from build123d import *

# Parameters (mm, degrees)
BOSS_EXTRU_1_DEPTH              = 12
ENL_V_MAT_EXTRU_1_DEPTH         = 119.989845505
ENL_V_MAT_EXTRU_2_DEPTH         = 11
ENL_V_MAT_EXTRU_3_DEPTH         = 9.5
BOSS_EXTRU_6_DEPTH              = 2.2
BOSS_EXTRU_8_DEPTH              = 1.5
BOSS_EXTRU_7_DEPTH              = 3
BOSS_EXTRU_7_DIRECTION_2_REACH  = 102.687
CHANFREIN3_SIZE                 = 2.2
ENL_V_DE_MAT_EXTRU_MINCE1_DEPTH = 1.6
ENL_V_DE_MAT_EXTRU_MINCE1_DRAFT = 10
ENL_V_MAT_EXTRU_10_DEPTH        = 11


with BuildPart() as part:
    # Esquisse1 → Boss.-Extru.1 (new body)
    with BuildSketch(Plane(origin=(0, 0, 0), x_dir=(1, 0, 0), z_dir=(0, 1, 0))):
        Polygon((-77.5, -44.744645862), (77.5, -44.744645862), (0, 89.489291724), align=None)
    extrude(amount=BOSS_EXTRU_1_DEPTH)

    # Esquisse2 → Enlèv. mat.-Extru.1 (cut, through all)
    with BuildSketch(Plane(origin=(0, 12, 0), x_dir=(1, 0, 0), z_dir=(0, 1, 0))):
        Polygon((-9.237604307, 73.489291724), (9.237604307, 73.489291724), (0, 89.489291724), align=None)
        Polygon((77.5, -44.744645862), (68.262395693, -28.744645862), (59.024791386, -44.744645862), align=None)
        Polygon((-77.5, -44.744645862), (25.833333333, -44.744645862), (-25.833333333, 44.744645862), align=None)
    extrude(amount=-ENL_V_MAT_EXTRU_1_DEPTH, mode=Mode.SUBTRACT)

    # Esquisse3 → Enlèv. mat.-Extru.2 (cut)
    with BuildSketch(Plane(origin=(0, 12, 0), x_dir=(1, 0, 0), z_dir=(0, 1, 0))):
        with BuildLine():
            Line((59.313466521, -20.244645862), (12.124355653, 61.489291724))
            ThreePointArc((12.124355653, 61.489291724), (0, 68.489291724), (-12.124355653, 61.489291724))
            Line((-12.124355653, 61.489291724), (-21.791881449, 44.744645862))
            Line((-21.791881449, 44.744645862), (27.854059275, -41.244645862))
            Line((27.854059275, -41.244645862), (47.189110868, -41.244645862))
            ThreePointArc((47.189110868, -41.244645862), (59.313466521, -34.244645862), (59.313466521, -20.244645862))
        make_face()
    extrude(amount=-ENL_V_MAT_EXTRU_2_DEPTH, mode=Mode.SUBTRACT)

    # Esquisse4 → Enlèv. mat.-Extru.3 (cut)
    with BuildSketch(Plane(origin=(0, 12, 0), x_dir=(1, 0, 0), z_dir=(0, 1, 0))):
        Polygon((37.068911087, 18.284054341), (34.368911087, 22.960591521), (37.4, 24.710591521), (40.1, 20.034054341), align=None)
    extrude(amount=-ENL_V_MAT_EXTRU_3_DEPTH, mode=Mode.SUBTRACT)

    # Esquisse14 → Boss.-Extru.6 (add)
    with BuildSketch(Plane(origin=(0, 1, 0), x_dir=(1, 0, 0), z_dir=(0, 1, 0))):
        Polygon((32.699295844, 24.65244995), (37.699295844, 15.992195912), (35.967245037, 14.992195912), (30.967245037, 23.65244995), align=None)
    extrude(amount=BOSS_EXTRU_6_DEPTH)

    # Esquisse19 → Boss.-Extru.8 (add)
    with BuildSketch(Plane(origin=(0, 2.5, 0), x_dir=(1, 0, 0), z_dir=(0, 1, 0))):
        Polygon((34.368911087, 22.960591521), (37.068911087, 18.284054341), (36.549295844, 17.984054341), (33.849295844, 22.660591521), align=None)
    extrude(amount=-BOSS_EXTRU_8_DEPTH)

    # Esquisse15 → Boss.-Extru.7 (add)
    with BuildSketch(Plane(origin=(0, 3.2, 0), x_dir=(1, 0, 0), z_dir=(0, 1, 0))):
        Polygon((35.159103466, 20.991938173), (35.759103466, 19.952707689), (33.767245037, 18.802707689), (33.167245037, 19.841938173), align=None)
    extrude(amount=BOSS_EXTRU_7_DEPTH)

    # Boss.-Extru.7 direction 2: up to this face of the body (flat: up to its plane)
    boss_extru_7_direction_2_end = Plane(part.part.faces().sort_by_distance((19.594473703, 1, -11.312874667))[0])
    # Esquisse15 → Boss.-Extru.7 direction 2 (add, up to the picked face)
    with BuildSketch(Plane(origin=(0, 3.2, 0), x_dir=(1, 0, 0), z_dir=(0, 1, 0)), mode=Mode.PRIVATE) as boss_extru_7_direction_2_sk1:
        Polygon((35.159103466, 20.991938173), (35.759103466, 19.952707689), (33.767245037, 18.802707689), (33.167245037, 19.841938173), align=None)
    boss_extru_7_direction_2_tool1 = split(extrude(boss_extru_7_direction_2_sk1.sketch, amount=-BOSS_EXTRU_7_DIRECTION_2_REACH, mode=Mode.PRIVATE), bisect_by=boss_extru_7_direction_2_end, keep=Keep.BOTH, mode=Mode.PRIVATE)
    add(boss_extru_7_direction_2_tool1.solids().sort_by(Axis((34.463174, 3.2, -19.897323), (0, -1, 0)))[0])

    # Chanfrein3
    chanfrein3_edges = [part.edges().sort_by_distance(p)[0] for p in [
        (33.467245037, 1, -19.322322931),
        (36.833270441, 1, -15.492195912),
        (31.833270441, 1, -24.15244995),
    ]]
    chamfer(chanfrein3_edges, length=CHANFREIN3_SIZE - 0.0001)  # a hair under: the kernel refuses the full size


with BuildPart() as enl_v_de_mat_extru_mince1_tool:
    # Esquisse17 → Enlèv. de mat.-Extru.-Mince1 (with draft: the straight prism first)
    with BuildSketch(Plane(origin=(0, 12, 0), x_dir=(1, 0, 0), z_dir=(0, 1, 0))):
        Polygon((37.4, 24.710591521), (9.237604307, 73.489291724), (-9.237604307, 73.489291724), (-25.833333333, 44.744645862), (25.833333333, -44.744645862), (59.024791386, -44.744645862), (68.262395693, -28.744645862), (40.1, 20.034054341), (38.454551733, 19.084054341), (66.06846467, -28.744645862), (57.927825874, -42.844645862), (26.930298845, -42.844645862), (-23.63940231, 44.744645862), (-8.140638796, 71.589291724), (8.140638796, 71.589291724), (35.754551733, 23.760591521), align=None)
    extrude(amount=-ENL_V_DE_MAT_EXTRU_MINCE1_DEPTH)
    # Enlèv. de mat.-Extru.-Mince1: the draft: its side faces are tilted about the plane it starts from
    enl_v_de_mat_extru_mince1_sides = [enl_v_de_mat_extru_mince1_tool.faces().sort_by_distance(p)[0] for p in [
        (23.318802154, 11.2, -49.099941623),
        (0, 11.2, -73.489291724),
        (-17.53546882, 11.2, -59.116968793),
        (0, 11.2, 0),
        (42.42906236, 11.2, 44.744645862),
        (63.643593539, 11.2, 36.744645862),
        (54.181197846, 11.2, 4.355295761),
        (39.277275866, 11.2, -19.559054341),
        (52.261508201, 11.2, 4.830295761),
        (61.998145272, 11.2, 35.794645862),
        (42.42906236, 11.2, 42.844645862),
        (1.645448267, 11.2, -0.95),
        (-15.890020553, 11.2, -58.166968793),
        (0, 11.2, -71.589291724),
        (21.947595264, 11.2, -47.674941623),
        (36.577275866, 11.2, -24.235591521),
    ]]
    draft(enl_v_de_mat_extru_mince1_sides, Plane(origin=(0, 12, 0), x_dir=(1, 0, 0), z_dir=(0, 1, 0)), ENL_V_DE_MAT_EXTRU_MINCE1_DRAFT)


with BuildPart() as part_1:
    add(part.part)

    # Enlèv. de mat.-Extru.-Mince1: cut by enl_v_de_mat_extru_mince1_tool
    add(enl_v_de_mat_extru_mince1_tool.part, mode=Mode.SUBTRACT)

    # Esquisse18 → Enlèv. mat.-Extru.10 (cut)
    with BuildSketch(Plane(origin=(0, 12, 0), x_dir=(1, 0, 0), z_dir=(0, 1, 0))):
        Polygon((57.613526329, -16.100263081), (59.518782217, -15.000263081), (54.268782217, -5.906996341), (52.363526329, -7.006996341), align=None)
        Polygon((20.113526329, 48.851642203), (14.863526329, 57.944908943), (16.768782217, 59.044908943), (22.018782217, 49.951642203), align=None)
    extrude(amount=-ENL_V_MAT_EXTRU_10_DEPTH, mode=Mode.SUBTRACT)


solid = part_1.part
Design review of the part built by this model. Coordinates are the model's own, in mm. A direction names the side the tool comes from. Coordinates: 2 decimals unless noted, no trailing zeros. Order: outer loops, then holes, each group sorted by start corner. A loop starts at its lowest first (then second) coordinate and runs counter-clockwise, first axis right, second up.
Item 1: For line 1 (Z direction, x = 15.5, y = 8.75); line 2 (Z direction, x = 57.5, y = 3.75); line 3 (X direction, y = 6.5, z = -52.5), list the stretches that pass through material, from the lowest coordinate up.
Item 2: For pin 1 Ø1 at (y, z) = (2.5, 4.5) entering from -X; pin 2 Ø1.8 at (x, z) = (35, -20) entering from +Y; pin 3 Ø3 at (y, z) = (5.5, -48) entering from -X, all flat-tipped, find the tip position at first contact; note any pin that passes through.
Item 3: Take a section at A-A, the plane y = 9. Write out the cut boundary in (x, z), then the cut area to 3 significant figures.
Item 4: Take a section at B-B, the plane x = 48.5. Write out the cut boundary in (y, z), then the cut area to 3 significant figures.
Item 5: For faces 4 (the flat face through (31, 10.4, -32)), 5 (the flat face through (28.14, 11.21, -36.67)), 6 (the flat face through (23.4, 6.58, -41.96)), list the 3-axis set-ups (+Z, -Z, +X, -X, +Y, -Y) from which the entire face can be reached by the end or side of a thin tool; tool diameter is ignored.
Item 6: Take a section at C-C, the plane z = 23. Write out the cut boundary in (x, y).
Item 7: The part is to be moulded in two halves that separate along Z. For faces 1 (the flat face through (31, 12, -31.6)), 2 (the flat face through (11.76, 11.21, -65.04)), 3 (the flat face through (2.684, 6.577, -2.352)), say which applies: pulls with the +Z half, pulls with the -Z half, needs draft (parallel to the pull), parting line crosses it, or undercut.
The answers:
1. line 1: z = -62.64 to -58.31, -56.84 to -55.64, 19.85 to 26.85
1. line 2: z = 10.1 to 11.5, 15.9 to 17.1, 36.71 to 44.74
1. line 3: x = -21.36 to -17.31, 17.31 to 18.01, 20.55 to 21.36
2. pin 1: stops at x = 2.31
2. pin 2: stops at y = 6.2
2. pin 3: stops at x = -24.82
3. outline: (-25.83, -44.74) - (-9.24, -73.49) - (9.24, -73.49) - (37.4, -24.71) - (34.37, -22.96) - (12.12, -61.49) arc R14 cw to (-12.12, -61.49) - (-21.79, -44.74) - (27.85, 41.24) - (47.19, 41.24) arc R14 cw to (59.31, 20.24) - (37.07, -18.28) - (40.1, -20.03) - (68.26, 28.74) - (59.02, 44.74) - (25.83, 44.74) - close; hole (14.86, -57.94) - (16.77, -59.04) - (22.02, -49.95) - (20.11, -48.85) - close; hole (52.36, 7.01) - (54.27, 5.91) - (59.52, 15) - (57.61, 16.1) - close
3. area: 1,120 mm2
4. outline: (0, -5.48) - (10.4, -5.48) - (10.4, -1.12) - (12, -1.68) - (12, 1.52) - (1, 1.52) - (1, 41.18) - (12, 41.18) - (12, 42.84) - (10.4, 42.56) - (10.4, 44.74) - (0, 44.74) - close
4. area: 157 mm2
5. face 4: none
5. face 5: -Z, +X
5. face 6: +Y
6. outline: (13.28, 0) - (64.95, 0) - (64.95, 10.4) - (62.43, 10.4) - (62.75, 12) - (60.53, 12) - (60.53, 1) - (17.32, 1) - (17.32, 12) - (15.47, 12) - (15.8, 10.4) - (13.28, 10.4) - close
7. face 1: needs draft
7. face 2: pulls with the -Z half
7. face 3: undercut
